```python
from build123d import *

# Parameters (mm, degrees)
SKETCH1_W           = 48
SKETCH1_H           = 46
SKETCH1_W_2         = 42.4
SKETCH1_H_2         = 40.4
BOSS_EXTRUDE1_DEPTH = 20
CUT_EXTRUDE1_REACH  = 59.498
SKETCH3_R           = 11.2
CUT_EXTRUDE2_REACH  = 59.498
SKETCH5_R           = 1.7
SKETCH6_W           = 8
SKETCH6_H           = 46
SKETCH6_R           = 2.25
SKETCH6_W_2         = 48
SKETCH6_H_2         = 8
BOSS_EXTRUDE2_DEPTH = 3
SKETCH7_R           = 3
CUT_EXTRUDE3_DEPTH  = 8


with BuildPart() as part:
    # Sketch1 → Boss-Extrude1 (new body)
    with BuildSketch(Plane.XY):
        with Locations((-4.106729999, -49.5)):
            Rectangle(SKETCH1_W, SKETCH1_H)
        with Locations((-4.106729999, -49.5)):
            Rectangle(SKETCH1_W_2, SKETCH1_H_2, mode=Mode.SUBTRACT)
    extrude(amount=-BOSS_EXTRUDE1_DEPTH)

    # Sketch3 → Cut-Extrude1 (cut, up to next)
    with BuildSketch(Plane(origin=(0, -26.5, 0), x_dir=(1, 0, 0), z_dir=(0, 1, 0)), mode=Mode.PRIVATE) as cut_extrude1_sk1:
        with Locations((-4.106729999, 21)):
            Circle(SKETCH3_R)
    cut_extrude1_tool1 = extrude(cut_extrude1_sk1.sketch, amount=-CUT_EXTRUDE1_REACH, mode=Mode.PRIVATE) & part.part
    add(cut_extrude1_tool1.solids().sort_by_distance((-4.10673, -26.5, -21))[0], mode=Mode.SUBTRACT)

    # Sketch5 → Cut-Extrude2 (cut, up to next)
    with BuildSketch(Plane(origin=(0, -26.5, 0), x_dir=(1, 0, 0), z_dir=(0, 1, 0)), mode=Mode.PRIVATE) as cut_extrude2_sk1:
        with Locations(Location((11.393270001, 5.5, 0), (0, 0, 270))):
            Circle(SKETCH5_R)
    cut_extrude2_tool1 = extrude(cut_extrude2_sk1.sketch, amount=-CUT_EXTRUDE2_REACH, mode=Mode.PRIVATE) & part.part
    # Sketch5 → Cut-Extrude2 (cut, up to next)
    with BuildSketch(Plane(origin=(0, -26.5, 0), x_dir=(1, 0, 0), z_dir=(0, 1, 0)), mode=Mode.PRIVATE) as cut_extrude2_sk2:
        with Locations(Location((-19.606729999, 5.5, 0), (0, 0, 270))):
            Circle(SKETCH5_R)
    cut_extrude2_tool2 = extrude(cut_extrude2_sk2.sketch, amount=-CUT_EXTRUDE2_REACH, mode=Mode.PRIVATE) & part.part
    add(cut_extrude2_tool1.solids().sort_by_distance((11.39327, -26.5, -5.5))[0], mode=Mode.SUBTRACT)
    add(cut_extrude2_tool2.solids().sort_by_distance((-19.60673, -26.5, -5.5))[0], mode=Mode.SUBTRACT)

    # Sketch6 → Boss-Extrude2 (add)
    # profile 1 of 2: a face of its own
    with BuildSketch(Plane.XY):
        with Locations((-32.106729999, -49.5)):
            Rectangle(SKETCH6_W, SKETCH6_H)
        with Locations((-32.106729999, -68.5)):
            Circle(SKETCH6_R, mode=Mode.SUBTRACT)
        with Locations((-32.106729999, -30.5)):
            Circle(SKETCH6_R, mode=Mode.SUBTRACT)
    # profile 2 of 2: a face of its own
    with BuildSketch(Plane.XY):
        with Locations((-4.106729999, -22.5)):
            Rectangle(SKETCH6_W_2, SKETCH6_H_2)
        with Locations((-24.106729999, -22.5)):
            Circle(SKETCH6_R, mode=Mode.SUBTRACT)
        with Locations((15.893270001, -22.5)):
            Circle(SKETCH6_R, mode=Mode.SUBTRACT)
    extrude(amount=-BOSS_EXTRUDE2_DEPTH)

    # Sketch7 → Cut-Extrude3 (cut)
    with BuildSketch(Plane(origin=(0, -18.5, 0), x_dir=(1, 0, 0), z_dir=(0, 1, 0))):
        with Locations((11.393270001, 5.5)):
            Circle(SKETCH7_R)
        with Locations((-19.606729999, 5.5)):
            Circle(SKETCH7_R)
    extrude(amount=-CUT_EXTRUDE3_DEPTH, mode=Mode.SUBTRACT)


solid = part.part
```
Source: CAD feature listing. Evaluate the final solid. Frame: model axes, mm. A direction names the side the tool comes from. Round coordinates to 2 decimals unless told otherwise and drop trailing zeros. Order: outer loops, then holes, each group sorted by start corner. A loop starts at its lowest first (then second) coordinate and runs counter-clockwise, first axis right, second up. Notation, with made-up numbers: (40.5, -22.5) -> (78.5, -22.5) arc R23 ccw to (78.5, -8.5) -> close; hole circle Ø5 at (-20.75, 68.5). An arc over 180 degrees is marked (long way). One line per item, written item: value. Start each with the question number.
Q1. Section query A-A (y = -68.5). Return the cut outline in (x, z).
Q2. Material intervals for probe 1 along X at (y, z) = (-27.55, -5.5); probe 2 along Y at (x, z) = (-14, -9.25); probe 3 along X at (y, z) = (-42, -10.25), sorted ascending.
Q3. Section query D-D (x = 4.5). Return the cut outline in (y, z), plus the area to 3 significant figures.
Q4. Section query C-C (z = -8.25). Return the cut outline in (x, y), plus the area to 3 significant figures.
Q5. Section query B-B (y = -53). Return the cut outline in (x, z), plus the area to 3 significant figures.
Q6. Pin query (flat end, axial travel): pin 1 (6 mm diameter, centred on x = -32.11, y = -30.5, fed in from +Z); pin 2 (2.5 mm diameter, centred on y = -23.5, z = -1.5, fed in from -X); pin 3 (4 mm diameter, centred on x = 12.5, z = -7, fed in from +Y); pin 4 (5 mm diameter, centred on x = 15.89, y = -22.5, fed in from -Z). Return the tip coordinate at first contact, or that it passes through.
Q7. Draft query along Y for faces 1 (the flat face through (-8, -72.5, -10)), 2 (the flat face through (-4, -29.3, -8)), 3 (the flat face through (-25.307, -50, -10)), 4 (the cylindrical face through (-4.3, -27.9, -9.8)). Return one class per face: pulls with the +Y half, pulls with the -Y half, needs draft (parallel to the pull), parting line crosses it, or undercut.
Q8. Access query for faces 5 (the cylindrical face through (-19.6, -22.4, -2.5)), 6 (the flat face through (-27, -39, 0)), 7 (the flat face through (-27, -22, -3)), 8 (the flat face through (-32, -49, -3)), 9 (the flat face through (-28.107, -23, -1)). Directions: +Z, -Z, +X, -X, +Y, -Y. A direction counts if a zero-diameter tool reaches every point of the face in a straight line with its end or side. Return the directions, or none.
Findings below:
1. outline: (-36.11, -3) -> (-34.36, -3) -> (-34.36, 0) -> (-36.11, 0) -> close; (-29.86, -3) -> (-28.11, -3) -> (-28.11, -20) -> (-25.31, -20) -> (-25.31, 0) -> (-29.86, 0) -> close; (17.09, -20) -> (19.89, -20) -> (19.89, 0) -> (17.09, 0) -> close
2. probe 1: -28.11 to -21.31, -17.91 to 9.69, 13.09 to 19.89
2. probe 2: -72.5 to -69.7, -29.3 to -26.5
2. probe 3: -28.11 to -25.31, 17.09 to 19.89
3. outline: (-72.5, -20) -> (-69.7, -20) -> (-69.7, 0) -> (-72.5, 0) -> close; (-29.3, -13.83) -> (-26.5, -13.83) -> (-26.5, -3) -> (-18.5, -3) -> (-18.5, 0) -> (-29.3, 0) -> close
3. area: 119 mm²
4. outline: (-28.11, -72.5) -> (19.89, -72.5) -> (19.89, -26.5) -> (-28.11, -26.5) -> close; hole (-25.31, -69.7) -> (17.09, -69.7) -> (17.09, -29.3) -> (-25.31, -29.3) -> close
4. area: 495 mm²
5. outline: (-36.11, -3) -> (-28.11, -3) -> (-28.11, -20) -> (-25.31, -20) -> (-25.31, 0) -> (-36.11, 0) -> close; (17.09, -20) -> (19.89, -20) -> (19.89, 0) -> (17.09, 0) -> close
5. area: 136 mm²
6. pin 1: z = 0
6. pin 2: x = -28.11
6. pin 3: y = -26.5
6. pin 4: z = -3
7. face 1: pulls with the -Y half
7. face 2: undercut
7. face 3: undercut
7. face 4: needs draft
8. face 5: -Z, +Y
8. face 6: +Z, +X, -X, +Y, -Y
8. face 7: -Z, +X, -X, +Y
8. face 8: -Z, -X, +Y, -Y
8. face 9: +Z, -Z, -X, +Y
